Input: part model. Units: mm. Frame: model coordinates. Face numbers are marked on the shaded views. A direction names the side the tool comes from. Round coordinates to 2 decimals unless told otherwise and drop trailing zeros. Loops run counter-clockwise (first coordinate to the right, second up) from the corner with the lowest first, then second, coordinate; pieces in that order, holes last. Notation, with made-up numbers: (82, -29.5) - (136, -29.5) arc R19 cw to (136, -17.5) - close; hole circle Ø9 at (-21.75, 39). An arc over 180 degrees is marked (long way). One line per question, with ' | ' between items. Start each with the question number.
Item 1: Draft query along Y for the marked faces 3, 4 and 5. Return one class per face: pulls with the +Y half, pulls with the -Y half, needs draft (parallel to the pull), parting line crosses it, or undercut.
Item 2: Section A-A, the plane y = -17. Return loops of the section in (x, z), plus the area to 3 significant figures.
Item 3: Material intervals for line 1 along X through (y, z) = (-45, -23.5); line 2 along Z through (x, y) = (39, -38.5); line 3 along Y through (x, z) = (-82, -9.75), sorted ascending.
Item 4: First-contact query: pin 1 (5 mm diameter, centred on x = -47, z = -4.5, fed in from +Y); pin 2 (1.2 mm diameter, centred on x = 59, z = -12.5, fed in from +Y). Flat tips, straight axial feed; report the tip coordinate or a pass-through.
Item 5: Section C-C, the plane x = 4.5. Return loops of the section in (y, z), plus the area to 3 significant figures.
Item 6: Section B-B, the plane z = -6. Return loops of the section in (x, y), plus the area to 4 significant figures.
Item 7: Set-up query: the marked faces 1 and 2. Return all of +Z, -Z, +X, -X, +Y, -Y with unobstructed straight access to the full face (end or side cutting, diameter ignored); none if empty.
Item 8: Section D-D, the plane y = -26.5. Return loops of the section in (x, z), plus the area to 3 significant figures.
```python
from build123d import *

# Parameters (mm, degrees)
F0_R          = 30
F2_DEPTH      = 5
F1_E0_TOP_W   = 150
F1_E0_TOP_H   = 25
F3_DEPTH      = 2.5
F5_E0_RIGHT_W = 75
F5_E0_RIGHT_H = 25
F6_DEPTH      = 2.5
F4_E0_LEFT_W  = 75
F4_E0_LEFT_H  = 25
F7_DEPTH      = 2.5


with BuildPart() as f2:
    # F0 (on Top) → F2 (new body)
    with BuildSketch(Plane.XY):
        with BuildLine():
            Line((54.8585835038, 26.6114953801), (-85.1414164962, 26.6114953801))
            ThreePointArc((-85.1414164962, 26.6114953801), (-88.6769504021, 25.1470292861), (-90.1414164962, 21.6114953801))
            Line((-90.1414164962, 21.6114953801), (-90.1414164962, -53.3885046199))
            Line((-90.1414164962, -53.3885046199), (59.8585835038, -53.3885046199))
            Line((59.8585835038, -53.3885046199), (59.8585835038, 21.6114953801))
            ThreePointArc((59.8585835038, 21.6114953801), (58.3941174097, 25.1470292861), (54.8585835038, 26.6114953801))
        make_face()
        with Locations((-50.1414164962, -13.3885046199)):
            Circle(F0_R, mode=Mode.SUBTRACT)
        with Locations((19.8585835038, -13.3885046199)):
            Circle(F0_R, mode=Mode.SUBTRACT)
    extrude(amount=F2_DEPTH)

    # F1_E0_top (on explicit) → F3 (join)
    with BuildSketch(Plane(origin=(-90.1414164962, -53.3885046199, 0), x_dir=(1, 0, 0), z_dir=(0, 1, 0))):
        with Locations((75, 12.5)):
            Rectangle(F1_E0_TOP_W, F1_E0_TOP_H)
    extrude(amount=F3_DEPTH)

    # F5_E0_right (on explicit) → F6 (join)
    with BuildSketch(Plane(origin=(59.8585835038, 21.6114953801, 0), x_dir=(0, -1, 0), z_dir=(1, 0, 0))):
        with Locations((37.5, 12.5)):
            Rectangle(F5_E0_RIGHT_W, F5_E0_RIGHT_H)
    extrude(amount=-F6_DEPTH)

    # F4_E0_left (on explicit) → F7 (join)
    with BuildSketch(Plane(origin=(-90.1414164962, 21.6114953801, 0), x_dir=(0, -1, 0), z_dir=(1, 0, 0))):
        with Locations((37.5, 12.5)):
            Rectangle(F4_E0_LEFT_W, F4_E0_LEFT_H)
    extrude(amount=F7_DEPTH)


solid = f2.part
```
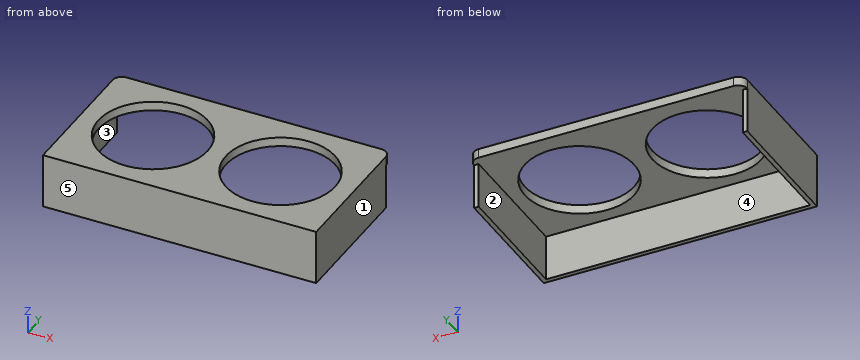
Return value:
1) face 3: needs draft | face 4: pulls with the +Y half | face 5: pulls with the -Y half
2) outline: (-90.14, -25) - (-87.64, -25) - (-87.64, 0) - (-79.92, 0) - (-79.92, 5) - (-90.14, 5) - close; (-20.36, 0) - (-9.92, 0) - (-9.92, 5) - (-20.36, 5) - close; (49.64, 0) - (57.36, 0) - (57.36, -25) - (59.86, -25) - (59.86, 5) - (49.64, 5) - close | area: 279 mm2
3) line 1: -90.14 to -87.64, 57.36 to 59.86 | line 2: 0 to 5 | line 3: -53.39 to -50.89
4) pin 1: y = -50.89 | pin 2: y = 21.61
5) outline: (-53.39, -25) - (-50.89, -25) - (-50.89, 0) - (-39.16, 0) - (-39.16, 5) - (-53.39, 5) - close; (12.38, 0) - (26.61, 0) - (26.61, 5) - (12.38, 5) - close | area: 205 mm2
6) outline: (-90.14, -53.39) - (59.86, -53.39) - (59.86, 21.61) - (57.36, 21.61) - (57.36, -50.89) - (-87.64, -50.89) - (-87.64, 21.61) - (-90.14, 21.61) - close | area: 737.5 mm2
7) face 1: +Z, -Z, +X, +Y, -Y | face 2: -Z, +Y
8) outline: (-90.14, -25) - (-87.64, -25) - (-87.64, 0) - (-77.12, 0) - (-77.12, 5) - (-90.14, 5) - close; (-23.16, 0) - (-7.12, 0) - (-7.12, 5) - (-23.16, 5) - close; (46.84, 0) - (57.36, 0) - (57.36, -25) - (59.86, -25) - (59.86, 5) - (46.84, 5) - close | area: 335 mm2
